from build123d import *

# Parameters (mm, degrees)
SALIENTE_EXTRUIR2_DEPTH = 15
SALIENTE_EXTRUIR3_DEPTH = 1.5
CROQUIS2_R              = 1.6
CORTAR_EXTRUIR1_DEPTH   = 10
CROQUIS4_R              = 4.5
SALIENTE_EXTRUIR4_DEPTH = 3.2
CORTAR_EXTRUIR2_REACH   = 42


with BuildPart() as part:
    # Croquis1 → Saliente-Extruir2 (new body)
    with BuildSketch(Plane.XY):
        with BuildLine():
            Line((51.828427125, 37), (6.178295218, 37))
            Line((6.178295218, 37), (0, 30.892284874))
            Line((0, 30.892284874), (0, 4.5))
            Line((0, 4.5), (-1.5, 4.5))
            Line((-1.5, 4.5), (-1.5, 2))
            Line((-1.5, 2), (0, 2))
            Line((0, 2), (0, 1))
            ThreePointArc((0, 1), (-0.292893219, 0.292893219), (-1, 0))
            Line((-1, 0), (-2, 0))
            ThreePointArc((-2, 0), (-2.707106781, 0.292893219), (-3, 1))
            Line((-3, 1), (-3, 30))
            ThreePointArc((-3, 30), (-2.603319545, 31.979386186), (-1.474544268, 33.65306221))
            Line((-1.474544268, 33.65306221), (3.484834866, 38.555786))
            ThreePointArc((3.484834866, 38.555786), (5.099859216, 39.624874593), (7, 40))
            Line((7, 40), (51, 40))
            ThreePointArc((51, 40), (52.913417162, 39.619397663), (54.535533906, 38.535533906))
            Line((54.535533906, 38.535533906), (59.535533906, 33.535533906))
            ThreePointArc((59.535533906, 33.535533906), (60.619397663, 31.913417162), (61, 30))
            Line((61, 30), (61, 1))
            ThreePointArc((61, 1), (60.707106781, 0.292893219), (60, 0))
            Line((60, 0), (59, 0))
            ThreePointArc((59, 0), (58.292893219, 0.292893219), (58, 1))
            Line((58, 1), (58, 2))
            Line((58, 2), (59.5, 2))
            Line((59.5, 2), (59.5, 4.5))
            Line((59.5, 4.5), (58, 4.5))
            Line((58, 4.5), (58, 30.828427125))
            Line((58, 30.828427125), (51.828427125, 37))
        make_face()
    extrude(amount=SALIENTE_EXTRUIR2_DEPTH)

    # Croquis3 → Saliente-Extruir3 (add)
    with BuildSketch(Plane.XY):
        Polygon((0, 27), (58, 27), (58, 30.828427125), (51.828427125, 37), (6.178295218, 37), (0, 30.892284874), align=None)
    extrude(amount=SALIENTE_EXTRUIR3_DEPTH)

    # Croquis2 → Cortar-Extruir1 (cut)
    with BuildSketch(Plane(origin=(0, 40, 0), x_dir=(1, 0, 0), z_dir=(0, 1, 0))):
        with Locations((9, -8)):
            Circle(CROQUIS2_R)
        with Locations((49, -8)):
            Circle(CROQUIS2_R)
    extrude(amount=-CORTAR_EXTRUIR1_DEPTH, mode=Mode.SUBTRACT)

    # Croquis4 → Saliente-Extruir4 (add)
    with BuildSketch(Plane.XZ.offset(-37)):
        with Locations((49, 8)):
            Circle(CROQUIS4_R)
        Polygon((52.05, 8), (50.525, 10.641377482), (47.475, 10.641377482), (45.95, 8), (47.475, 5.358622518), (50.525, 5.358622518), align=None, mode=Mode.SUBTRACT)
        with Locations((9, 8)):
            Circle(CROQUIS4_R)
        Polygon((10.525, 10.641377482), (7.475, 10.641377482), (5.95, 8), (7.475, 5.358622518), (10.525, 5.358622518), (12.05, 8), align=None, mode=Mode.SUBTRACT)
    extrude(amount=SALIENTE_EXTRUIR4_DEPTH)

    # Croquis5 → Cortar-Extruir2 (cut, up to next)
    with BuildSketch(Plane(origin=(0, 40, 0), x_dir=(1, 0, 0), z_dir=(0, 1, 0)), mode=Mode.PRIVATE) as cortar_extruir2_sk1:
        with BuildLine():
            Line((9.275661815, -15), (48.724338185, -15))
            ThreePointArc((48.724338185, -15), (29, -5.360679775), (9.275661815, -15))
        make_face()
    cortar_extruir2_tool1 = extrude(cortar_extruir2_sk1.sketch, amount=-CORTAR_EXTRUIR2_REACH, mode=Mode.PRIVATE) & part.part
    add(cortar_extruir2_tool1.solids().sort_by_distance((29, 40, 11.072485))[0], mode=Mode.SUBTRACT)


solid = part.part
Source: CAD feature listing. Evaluate the final solid. Frame: model axes, mm. A direction names the side the tool comes from. Coordinates: 2 decimals unless noted, no trailing zeros. Loops run counter-clockwise (first coordinate to the right, second up) from the corner with the lowest first, then second, coordinate; pieces in that order, holes last. Notation, with made-up numbers: (19, -22.5) - (40, -22.5) arc R19 cw to (40, -12.5) - close; hole circle Ø9 at (50.25, 48). An arc over 180 degrees is marked (long way). Return JSON: item names as keys, results as strings.
Q1. Section D-D, the plane y = 16. Return loops of the section in (x, z), plus the area to 3 significant figures.
Results:
{"outline": "(-3, 0) - (0, 0) - (0, 15) - (-3, 15) - close; (58, 0) - (61, 0) - (61, 15) - (58, 15) - close", "area": "90.0 mm2"}
Q2. Section A-A, the plane y = 3. Return loops of the section in (x, z), plus the area to 3 significant figures.
Results:
{"outline": "(-3, 0) - (-1.5, 0) - (-1.5, 15) - (-3, 15) - close; (59.5, 0) - (61, 0) - (61, 15) - (59.5, 15) - close", "area": "45.0 mm2"}
Q3. Section C-C, the plane z = 2.5. Return loops of the section in (x, y).
Results:
{"outline": "(-3, 1) arc R1 ccw to (-2, 0) - (-1, 0) arc R1 ccw to (0, 1) - (0, 2) - (-1.5, 2) - (-1.5, 4.5) - (0, 4.5) - (0, 30.89) - (6.18, 37) - (51.83, 37) - (58, 30.83) - (58, 4.5) - (59.5, 4.5) - (59.5, 2) - (58, 2) - (58, 1) arc R1 ccw to (59, 0) - (60, 0) arc R1 ccw to (61, 1) - (61, 30) arc R5 ccw to (59.54, 33.54) - (54.54, 38.54) arc R5 ccw to (51, 40) - (7, 40) arc R5 ccw to (3.48, 38.56) - (-1.47, 33.65) arc R5.14 ccw to (-3, 30) - close"}
Q4. Contact query for flat-ended pins moving along their axis: P1, Ø2.5, axis at x = 48, z = 7.5, coming from the -Y side; P2, Ø0.8, axis at x = 32.5, z = 0.5, coming from the -Y side; P3, Ø5, axis at y = 33, z = 7.5, coming from the +X side. Output: stop coordinate, or through.
Results:
{"P1": "y = 37", "P2": "y = 27", "P3": "x = 60.97"}
Q5. Access query for faces 1 (the cylindrical face through (52.89, 39.63, 7.4)), 2 (the flat face through (9, 33.8, 5)), 3 (the flat face through (49, 35, 10.641)), 4 (the flat face through (59.5, 3, 7)), 5 (the cylindrical face through (-2.614, 31.953, 7.395)). Directions: +Z, -Z, +X, -X, +Y, -Y. A direction counts if a zero-diameter tool reaches every point of the face in a straight line with its end or side. Return the directions, or none.
Results:
{"face 1": "+Z, -Z, +X, +Y", "face 2": "+Z, -Y", "face 3": "-Y", "face 4": "+Z, -Z", "face 5": "+Z, -Z, -X, +Y"}
Q6. Mould query, pull axis Z, two halves, no side actions, for faces 6 (the flat face through (-1.5, 3, 7)), 7 (the cylindrical face through (29.318, 38.521, 5.363)), 8 (the flat face through (6.7, 35.4, 6.7)). Classes: released by +Z, released by -Z, zero draft, split by the parting line, or undercut.
Results:
{"face 6": "zero draft", "face 7": "released by +Z", "face 8": "undercut"}
Q7. Section B-B, the plane y = 36. Return loops of the section in (x, z) (3 decimals).
Results:
{"outline": "(0.9, 0) - (57.071, 0) - (57.071, 15) - (52.828, 15) - (52.828, 10.365) arc R4.5 ccw (long way) to (52.828, 5.635) - (52.828, 1.5) - (5.167, 1.5) - (5.167, 5.643) arc R4.5 ccw (long way) to (5.167, 10.357) - (5.167, 15) - (0.9, 15) - close; hole (5.95, 8) - (7.475, 5.359) - (10.525, 5.359) - (12.05, 8) - (10.525, 10.641) - (7.475, 10.641) - close; hole (45.95, 8) - (47.475, 5.359) - (50.525, 5.359) - (52.05, 8) - (50.525, 10.641) - (47.475, 10.641) - close"}
Q8. Material intervals for line 1 along X through (y, z) = (10, 4.25); line 2 along Z through (x, y) = (9, 38.05); line 3 along X through (y, z) = (38.4, 8), sorted ascending.
Results:
{"line 1": "-3 to 0, 58 to 61", "line 2": "0 to 6.4, 9.6 to 15", "line 3": "3.33 to 7.4, 10.6 to 17.82, 40.18 to 47.4, 50.6 to 54.67"}
